Autodesk Inventor part; units mm, degrees
ref_plane "YZ Plane" through (0, 0, 0) normal (1, 0, 0) x (0, 1, 0)
ref_plane "XZ Plane" through (0, 0, 0) normal (0, 1, 0) x (-1, 0, 0)
ref_plane "XY Plane" through (0, 0, 0) normal (0, 0, 1) x (1, 0, 0)
sketch "Sketch1" plane through (0, 0, 0) normal (0, 0, 1) x (1, 0, 0)
  line L0 (6.4984, 1.7965) -> (6.4984, 46.7965)
  line L1 (6.4984, 1.7965) -> (343.9984, 1.7965)
  line L2 (343.9984, 1.7965) -> (343.9984, 36.7965)
  line L3 (343.9984, 36.7965) -> (6.4984, 46.7965)
  line L4 (6.4984, 46.7965) -> (6.4984, 76.7965)
  line L5 (6.4984, 76.7965) -> (343.9984, 76.7965)
  line L6 (343.9984, 76.7965) -> (343.9984, 36.7965)
  line L7 (6.4984, 76.7965) -> (1.4984, 76.7965)
  line L8 (1.4984, 76.7965) -> (1.4984, 1.7965)
  line L9 (1.4984, 1.7965) -> (6.4984, 1.7965)
  point P0 (0, 0)
  dimension "d0" = 45
  dimension "d1" = 35
  dimension "d2" = 337.5
  dimension "d3" = 30
  dimension "d12" = 5
extrude "Extrusion1" add sketch "Sketch1" against normal blind 45 contours L0 L3 L2 L1
extrude "Extrusion3" add sketch "Sketch1" against normal blind 5 contours L4 L5 L6 L3
extrude "Extrusion5" add sketch "Sketch1" against normal blind 45 contours L9 L8 L7 L4 L0
properties part number "collectingslide"
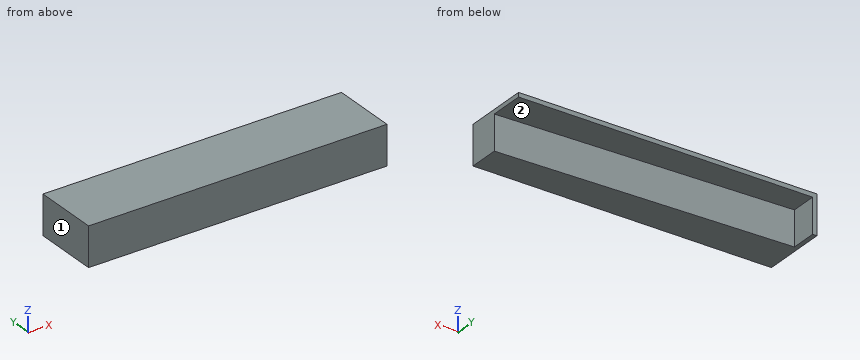
Could you check a few things on this model? Use its own coordinates, in mm. Face numbers are marked on the shaded views. A direction names the side the tool comes from. Round coordinates to 2 decimals unless told otherwise and drop trailing zeros. Order: outer loops, then holes, each group sorted by start corner. A loop starts at its lowest first (then second) coordinate and runs counter-clockwise, first axis right, second up. Notation, with made-up numbers: (-27, 82) -> (17, 82) arc R6 cw to (17, 93) -> close; hole circle Ø11 at (22, 65.5). An arc over 180 degrees is marked (long way). One line per question, with ' | ' between items.
Q1. If I drill on line 1 (Z direction, x = 239.5, y = 66); line 2 (X direction, y = 73, z = -24); line 3 (Y direction, x = 37.5, z = -9), over which ranges is the centre line in solid material (lowest first)? Write a range as from..to.
Computed values:
line 1: -5..0 | line 2: 1.5..6.5 | line 3: 1.8..45.88
Q2. If we section it at B-B on z = -23: Write out the boundary of the cut face in (x, y).
Computed values:
outline: (1.5, 1.8) -> (344, 1.8) -> (344, 36.8) -> (6.5, 46.8) -> (6.5, 76.8) -> (1.5, 76.8) -> close
Q3. I'm going to push flat-ended pins straight in: pin 1 (10 mm diameter, centred on x = 90, z = -29, fed in from +Y); pin 2 (12 mm diameter, centred on x = 161.5, y = 52, fed in from -Z); pin 3 (1.5 mm diameter, centred on y = 59, z = -29, fed in from +X). Where does each tip first touch, or does it pass through?
Computed values:
pin 1: y = 44.47 | pin 2: z = -5 | pin 3: x = 6.5
Q4. If we section it at A-A on y = 68.5: Write out the boundary of the cut face in (x, z).
Computed values:
outline: (1.5, -45) -> (6.5, -45) -> (6.5, -5) -> (344, -5) -> (344, 0) -> (1.5, 0) -> close
Q5. Which directions (+Z, -Z, +X, -X, +Y, -Y) give clear straight access to the entire face, cutting with the end or side of a thin tool? Please do the marked faces 1 and 2.
Computed values:
face 1: +Z, -Z, -X, +Y, -Y | face 2: -Z, +X, +Y
